from build123d import *

# Parameters (mm, degrees)
SKETCH006_W                = 25.4
SKETCH006_H                = 25.4
PAD005_DEPTH               = 1.6
SKETCH005_R                = 1.778
POCKET_DEPTH               = 73.514281
SKETCH005_MIRRORED006_2_R  = 1.778
POCKET_MIRRORED006_2_DEPTH = 73.514281


with BuildPart() as part:
    # Sketch006 → Pad005 (new body)
    with BuildSketch(Plane.XY):
        Rectangle(SKETCH006_W, SKETCH006_H)
    extrude(amount=PAD005_DEPTH)

    # Sketch005 (on Face6 of Pad005) → Pocket (cut, through all)
    with BuildSketch(Plane.XY.offset(1.6)):
        with Locations((-10.16, 10.16)):
            Circle(SKETCH005_R)
    pocket = extrude(amount=-POCKET_DEPTH, mode=Mode.SUBTRACT)

    # Sketch005 Mirrored006 2 → Pocket Mirrored006 2 (cut, through all)
    with BuildSketch(Plane(origin=(0, 0, 1.6), x_dir=(-1, 0, 0), z_dir=(0, 0, -1))):
        with Locations((-10.16, 10.16)):
            Circle(SKETCH005_MIRRORED006_2_R)
    pocket_mirrored006_2 = extrude(amount=POCKET_MIRRORED006_2_DEPTH, mode=Mode.SUBTRACT)

    # Mirrored007: Pocket, Pocket Mirrored006 2 across XZ
    add(pocket.mirror(Plane.XZ), mode=Mode.SUBTRACT)
    add(pocket_mirrored006_2.mirror(Plane.XZ), mode=Mode.SUBTRACT)


solid = part.part
CAD build for the part. Positions are in the model's coordinates, mm. Coordinates: 2 decimals unless noted, no trailing zeros. Write each loop counter-clockwise with the first axis right and the second up, starting at its lowest first coordinate (ties: lowest second). Pieces come first, ordered by that corner, then holes. Notation, with made-up numbers: (-17.75, 35) - (-12.75, 35) arc R30 cw to (-12.75, 69) - close; hole circle Ø6 at (59.25, 15). An arc over 180 degrees is marked (long way). Use a Markdown table: item, result. Add a question column.
Item 1: Band-saw the part on B-B, the plane z = 0.5. Give the cut face in (x, y), and give its area (3 significant figures).
Item 2: Mould opens along X. For faces 1 (the face through (-11.47, -11.36, 0.81)), 2 (the face through (11.47, 11.36, 0.81)), 3 (the face through (-12.7, 0, 1)), 4 (the face through (0, 12.7, 1)) say: pulls with the +X half, pulls with the -X half, needs draft (parallel to the pull), parting line crosses it, or undercut.
Item 3: Flat gauge pin, fed straight in: pin 1 (1 mm diameter, centred on x = -9.5, y = -2, fed in from -Z). Where does the tip first touch, or does it go through?
Item 4: Drill centre lines: L1, parallel to X at y = -10, z = 0.2; L2, parallel to Y at x = -10.16, z = 1.1; L3, parallel to X at y = -9.5, z = 0.1. Where is each one in solid material? Low to high. Write a range as from..to.
Item 5: Band-saw the part on A-A, the plane y = -10.16. Give the cut face in (x, z), and give its area (3 significant figures).
Numbers:
| question | item | result |
|---|---|---|
| 1 | outline | (-12.7, -12.7) - (12.7, -12.7) - (12.7, 12.7) - (-12.7, 12.7) - close; hole circle Ø3.56 at (-10.16, -10.16); hole circle Ø3.56 at (-10.16, 10.16); hole circle Ø3.56 at (10.16, -10.16); hole circle Ø3.56 at (10.16, 10.16) |
| 1 | area | 605 mm2 |
| 2 | face 1 | undercut |
| 2 | face 2 | undercut |
| 2 | face 3 | pulls with the -X half |
| 2 | face 4 | needs draft |
| 3 | pin 1 | z = 0 |
| 4 | L1 | -12.7..-11.93, -8.39..8.39, 11.93..12.7 |
| 4 | L2 | -12.7..-11.94, -8.38..8.38, 11.94..12.7 |
| 4 | L3 | -12.7..-11.81, -8.51..8.51, 11.81..12.7 |
| 5 | outline | (-12.7, 0) - (-11.94, 0) - (-11.94, 1.6) - (-12.7, 1.6) - close; (-8.38, 0) - (8.38, 0) - (8.38, 1.6) - (-8.38, 1.6) - close; (11.94, 0) - (12.7, 0) - (12.7, 1.6) - (11.94, 1.6) - close |
| 5 | area | 29.3 mm2 |
